Can you work these out from the model? Positions are in its coordinate system, mm. Face numbers are marked on the shaded views. A direction names the side the tool comes from. Coordinates: 2 decimals unless noted, no trailing zeros. Order: outer loops, then holes, each group sorted by start corner. A loop starts at its lowest first (then second) coordinate and runs counter-clockwise, first axis right, second up. Notation, with made-up numbers: (44.25, 58) -> (48.25, 58) arc R26 cw to (48.25, 90) -> close; hole circle Ø1 at (9, 50.5). An arc over 180 degrees is marked (long way). Write item = value, one per line.
```python
from build123d import *

# Parameters (mm, degrees)
SKETCH_2_R          = 2
CUT_EXTRUDE_1_DEPTH = 2.5
SKETCH_3_R          = 3.6
CUT_EXTRUDE_2_DEPTH = 2.5
SKETCH_4_R          = 4.3
CUT_EXTRUDE_3_DEPTH = 0.8


with BuildPart() as part:
    # 스케치1 → 회전1 (revolve)
    with BuildSketch(Plane.XY):
        Polygon((0, 0), (0, 2.5), (-7.5, 2.5), (-6.5, 1.25), (-7.5, 0), align=None)
    revolve(axis=Axis((0, 2.5, 0), (0, -1, 0)))

    # 스케치2 → 컷-돌출1 (cut)
    with BuildSketch(Plane(origin=(0, 2.5, 0), x_dir=(1, 0, 0), z_dir=(0, 1, 0))):
        Circle(SKETCH_2_R)
    extrude(amount=-CUT_EXTRUDE_1_DEPTH, mode=Mode.SUBTRACT)

    # 스케치3 → 컷-돌출2 (cut)
    with BuildSketch(Plane(origin=(0, 2.5, 0), x_dir=(1, 0, 0), z_dir=(0, 1, 0))):
        Circle(SKETCH_3_R)
    extrude(amount=-CUT_EXTRUDE_2_DEPTH, mode=Mode.SUBTRACT)

    # 스케치4 → 컷-돌출3 (cut)
    with BuildSketch(Plane(origin=(0, 2.5, 0), x_dir=(1, 0, 0), z_dir=(0, 1, 0))):
        Circle(SKETCH_4_R)
    extrude(amount=-CUT_EXTRUDE_3_DEPTH, mode=Mode.SUBTRACT)


solid = part.part
```
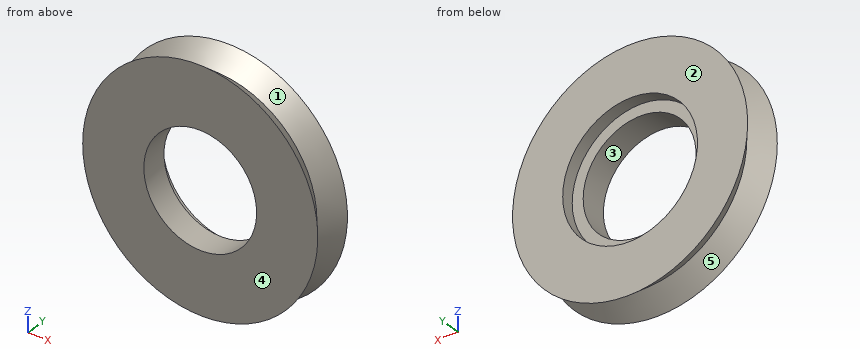
Item 1: If we mould it in two halves opening along Y, with no side actions, what happens to the marked faces 1, 2 and 3? For each: pulls with the +Y half, pulls with the -Y half, needs draft (parallel to the pull), parting line crosses it, or undercut.
A:
face_1 = undercut
face_2 = pulls with the +Y half
face_3 = needs draft
Item 2: I'm going to push flat-ended pins straight in: P1, Ø7.5, axis at x = 0, z = 0, coming from the -Y side; P2, Ø1, axis at x = -2.5, y = 2, coming from the +Z side; P3, Ø6.5, axis at x = 0, z = 0, coming from the -Y side; P4, Ø4, axis at x = 1.5, z = -1, coming from the +Y side. Where does each tip first touch, or does it pass through?
A:
P1 = 0
P2 = 7.1
P3 = through
P4 = 1.7
Item 3: I want a section at A-A, the plane x = 0. Please give me the cut outline in (y, z), plus the area to 3 significant figures.
A:
outline = (0, -7.5) -> (1.25, -6.5) -> (2.5, -7.5) -> (2.5, -4.3) -> (1.7, -4.3) -> (1.7, -3.6) -> (0, -3.6) -> close; (0, 3.6) -> (1.7, 3.6) -> (1.7, 4.3) -> (2.5, 4.3) -> (2.5, 7.5) -> (1.25, 6.5) -> (0, 7.5) -> close
area = 15.9 mm2
Item 4: If I drill on probe 1 along X at (y, z) = (2.1, 0); probe 2 along Z at (x, y) = (2.5, 1.55); probe 3 along X at (y, z) = (1.95, -1.25), over which ranges is the centre line in solid material (lowest first)?
A:
probe_1 = -7.18 to -4.3, 4.3 to 7.18
probe_2 = -6.26 to -2.59, 2.59 to 6.26
probe_3 = -6.95 to -4.11, 4.11 to 6.95
Item 5: For the marked faces 4 and 5, which set-ups out of +Z, -Z, +X, -X, +Y, -Y let a thin tool reach every point of the face, with its end or its side?
A:
face_4 = +Z, -Z, +X, -X, -Y
face_5 = none
Item 6: I want a section at C-C, the plane y = 2.2. Please give me the cut outline in (x, z).
A:
outline = circle Ø14.52 at (0, 0); hole circle Ø8.6 at (0, 0)
Item 7: I want a section at B-B, the plane y = 1.05. Please give me the cut outline in (x, z).
A:
outline = circle Ø13.32 at (0, 0); hole circle Ø7.2 at (0, 0)
